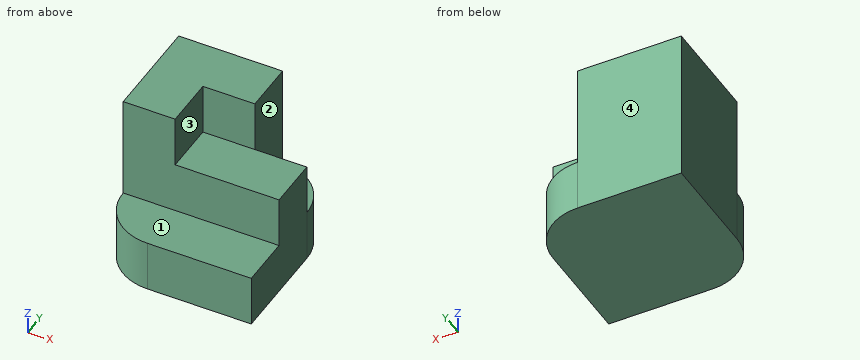
```python
from build123d import *

# Parameters (mm, degrees)
F0_W     = 25.4
F0_H     = 25.4
F1_DEPTH = 76.2
F2_DEPTH = 50.8
F3_DEPTH = 25.4


with BuildPart() as f1:
    # F0 (on Top) → F1 (new body)
    with BuildSketch(Plane.XY):
        with Locations((12.7, 63.5)):
            Rectangle(F0_W, F0_H)
        with BuildLine():
            ThreePointArc((25.4, 50.8), (7.4394877579, 43.3605122421), (0, 25.4))
            Line((0, 25.4), (25.4, 25.4))
            Line((25.4, 25.4), (25.4, 50.8))
        make_face()
        with BuildLine():
            Line((0, 50.8), (0, 25.4))
            ThreePointArc((0, 25.4), (7.4394877579, 43.3605122421), (25.4, 50.8))
            Line((25.4, 50.8), (0, 50.8))
        make_face()
        with BuildLine():
            ThreePointArc((50.8, 76.2), (32.8394877579, 68.7605122421), (25.4, 50.8))
            Line((25.4, 50.8), (50.8, 50.8))
            Line((50.8, 50.8), (50.8, 76.2))
        make_face()
        with BuildLine():
            Line((25.4, 76.2), (25.4, 50.8))
            ThreePointArc((25.4, 50.8), (32.8394877579, 68.7605122421), (50.8, 76.2))
            Line((50.8, 76.2), (25.4, 76.2))
        make_face()
    extrude(amount=F1_DEPTH)

    # F0 (on Top) → F2 (join)
    with BuildSketch(Plane.XY):
        with BuildLine():
            ThreePointArc((25.4, 50.8), (43.3605122421, 43.3605122421), (50.8, 25.4))
            Line((50.8, 25.4), (50.8, 50.8))
            Line((50.8, 50.8), (25.4, 50.8))
        make_face()
        with BuildLine():
            ThreePointArc((25.4, 50.8), (32.8394877579, 32.8394877579), (50.8, 25.4))
            ThreePointArc((50.8, 25.4), (43.3605122421, 43.3605122421), (25.4, 50.8))
        make_face()
        with BuildLine():
            Line((25.4, 50.8), (25.4, 25.4))
            Line((25.4, 25.4), (50.8, 25.4))
            ThreePointArc((50.8, 25.4), (32.8394877579, 32.8394877579), (25.4, 50.8))
        make_face()
        with BuildLine():
            Line((50.8, 50.8), (50.8, 25.4))
            ThreePointArc((50.8, 25.4), (68.7605122421, 32.8394877579), (76.2, 50.8))
            Line((76.2, 50.8), (50.8, 50.8))
        make_face()
        with BuildLine():
            ThreePointArc((76.2, 50.8), (68.7605122421, 32.8394877579), (50.8, 25.4))
            Line((50.8, 25.4), (76.2, 25.4))
            Line((76.2, 25.4), (76.2, 50.8))
        make_face()
    extrude(amount=F2_DEPTH)

    # F0 (on Top) → F3 (join)
    with BuildSketch(Plane.XY):
        with Locations((63.5, 12.7)):
            Rectangle(F0_W, F0_H)
        with BuildLine():
            Line((25.4, 25.4), (25.4, 0))
            ThreePointArc((25.4, 0), (43.3605122421, 7.4394877579), (50.8, 25.4))
            Line((50.8, 25.4), (25.4, 25.4))
        make_face()
        with BuildLine():
            ThreePointArc((50.8, 25.4), (43.3605122421, 7.4394877579), (25.4, 0))
            Line((25.4, 0), (50.8, 0))
            Line((50.8, 0), (50.8, 25.4))
        make_face()
        with BuildLine():
            Line((50.8, 76.2), (50.8, 50.8))
            Line((50.8, 50.8), (76.2, 50.8))
            ThreePointArc((76.2, 50.8), (68.7605122421, 68.7605122421), (50.8, 76.2))
        make_face()
        with BuildLine():
            ThreePointArc((0, 25.4), (7.4394877579, 7.4394877579), (25.4, 0))
            Line((25.4, 0), (25.4, 25.4))
            Line((25.4, 25.4), (0, 25.4))
        make_face()
    extrude(amount=F3_DEPTH)


solid = f1.part
```
The model under review builds one solid part; all positions refer to its coordinate system, in mm. Face numbers are marked on the shaded views. A direction names the side the tool comes from. Round coordinates to 2 decimals unless told otherwise and drop trailing zeros. Order: outer loops, then holes, each group sorted by start corner. A loop starts at its lowest first (then second) coordinate and runs counter-clockwise, first axis right, second up. Notation, with made-up numbers: (85.5, -16) -> (103.5, -16) arc R4 cw to (103.5, -9) -> close; hole circle Ø7 at (-2.5, 76.25). An arc over 180 degrees is marked (long way). One line per item, written item: value. Start each with the question number.
Q1. Take a section at A-A (z = 12.5). Write out the cut boundary in (x, y).
Q2. Take a section at B-B (x = 59). Write out the cut boundary in (y, z).
Q3. Take a section at C-C (y = 48). Write out the cut boundary in (x, z).
Q4. Wall thickness on line 1 (X direction, y = 62.5, z = 30); line 2 (Z direction, x = 69, y = 13): over which ranges is each line inside the solid? List them lowest first.
Q5. Machinability: for the marked faces 1, 2, 3 and 4, which of the approach directions +Z, -Z, +X, -X, +Y, -Y give a long, thin tool a straight path to every point of the face, cutting with its end or side? Answer none if there is none.
Q6. Take a section at D-D (x = 38). Write out the cut boundary in (y, z), and give its area (3 significant figures).
Q7. Clearance check with flat-ended pins moving along their axes: pin 1 Ø20.5 at (x, y) = (52, 17) entering from +Z; pin 2 Ø8 at (x, z) = (18, 18) entering from -Y; pin 3 Ø10 at (x, z) = (47.5, 37.5) entering from -Y; pin 4 Ø12 at (x, y) = (28.5, 27.5) entering from +Z. State where each tip first meets the part, or that it passes through.
Reported:
1. outline: (0, 25.4) arc R25.4 ccw to (25.4, 0) -> (76.2, 0) -> (76.2, 50.8) arc R25.4 ccw to (50.8, 76.2) -> (0, 76.2) -> close
2. outline: (0, 0) -> (74.84, 0) -> (74.84, 25.4) -> (50.8, 25.4) -> (50.8, 50.8) -> (25.4, 50.8) -> (25.4, 25.4) -> (0, 25.4) -> close
3. outline: (0, 0) -> (76.2, 0) -> (76.2, 50.8) -> (25.4, 50.8) -> (25.4, 76.2) -> (0, 76.2) -> close
4. line 1: x = 0 to 50.8
4. line 2: z = 0 to 25.4
5. face 1: +Z, +X, -X, -Y
5. face 2: +Z, +X, +Y
5. face 3: +Z, +X, -Y
5. face 4: +Z, -Z, +X, -X, +Y
6. outline: (0, 0) -> (76.2, 0) -> (76.2, 76.2) -> (50.8, 76.2) -> (50.8, 50.8) -> (25.4, 50.8) -> (25.4, 25.4) -> (0, 25.4) -> close
6. area: 3,870 mm2
7. pin 1: stops at z = 50.8
7. pin 2: stops at y = 0.23
7. pin 3: stops at y = 25.4
7. pin 4: stops at z = 76.2
